Job drawing, mm, ordinate dimensions from the low corner. One solid piece. Round coordinates to 2 decimals unless told otherwise and drop trailing zeros. Write each loop counter-clockwise with the first axis right and the second up, starting at its lowest first coordinate (ties: lowest second). Pieces come first, ordered by that corner, then holes.
1) Pull direction X, two halves, no side cores. Call the marked faces 1, 2 and 3: +X half, -X half, draft (parallel to the pull), parting line (faces both ways), or undercut.
2) Saw through at A-A (y = 15). Write the cut outline in (x, z).
3) Saw through at D-D (x = 139). Write the cut outline in (y, z).
4) Saw through at B-B (z = 12.25). Write the cut outline in (x, y).
5) Wall check: probe 1 along X at (y, z) = (2.75, 12.5); probe 2 along X at (y, z) = (12, 1); probe 3 along Y at (x, z) = (163, 9.25). Give the ranges that are in metal, low to high.
6) Saw through at C-C (z = 4). Write the cut outline in (x, y).
7) Flat gauge pins, fed straight in: pin 1 (10 mm diameter, centred on x = 90, z = 7, fed in from +Y); pin 2 (5 mm diameter, centred on x = 115, y = 3, fed in from +Z). Where does each tip first touch, or does it go through?
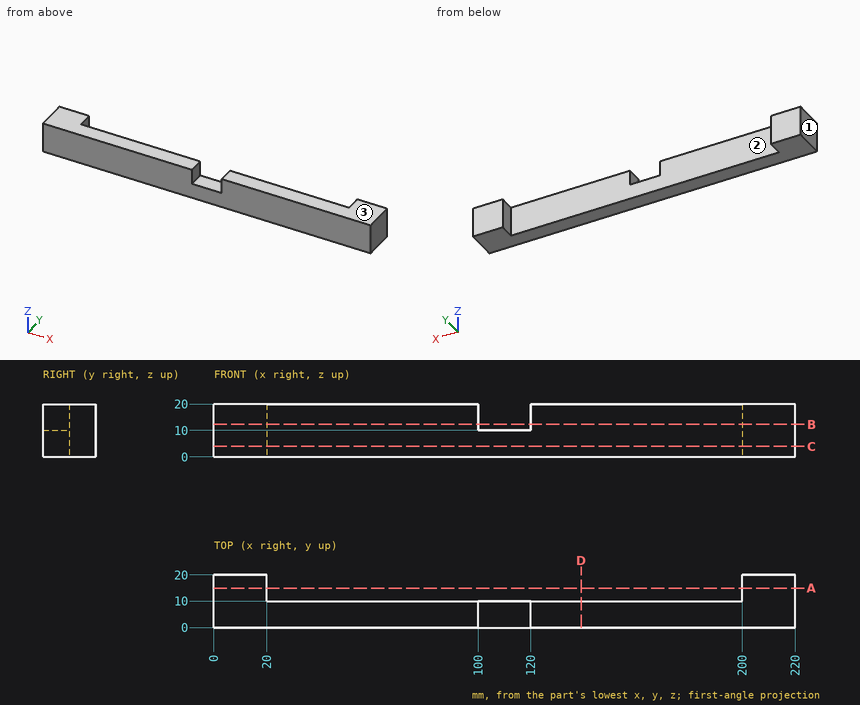
Evaluation:
1. face 1: -X half
1. face 2: undercut
1. face 3: draft
2. outline: (0, 0) - (20, 0) - (20, 20) - (0, 20) - close; (200, 0) - (220, 0) - (220, 20) - (200, 20) - close
3. outline: (0, 0) - (10, 0) - (10, 20) - (0, 20) - close
4. outline: (0, 0) - (100, 0) - (100, 10) - (20, 10) - (20, 20) - (0, 20) - close; (120, 0) - (220, 0) - (220, 20) - (200, 20) - (200, 10) - (120, 10) - close
5. probe 1: x = 0 to 100, 120 to 220
5. probe 2: x = 0 to 20, 200 to 220
5. probe 3: y = 0 to 10
6. outline: (0, 0) - (220, 0) - (220, 20) - (200, 20) - (200, 10) - (20, 10) - (20, 20) - (0, 20) - close
7. pin 1: stops at y = 10
7. pin 2: stops at z = 10
